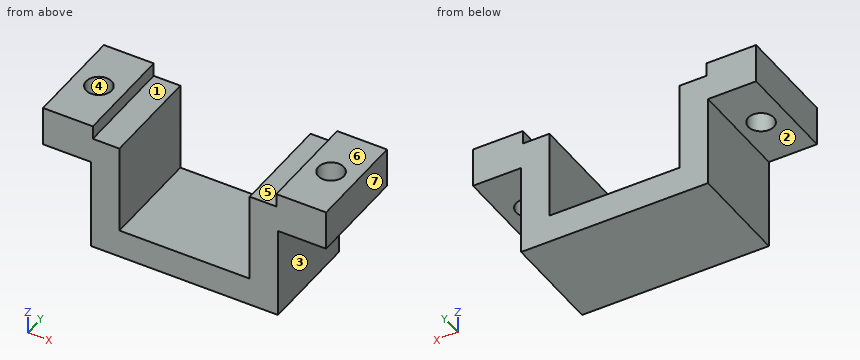
```python
from build123d import *

# Parameters (mm, degrees)
BOSS_EXTRUDE1_DEPTH = 18
SKETCH2_R           = 2.25
CUT_EXTRUDE1_DEPTH  = 56.555737777


with BuildPart() as part:
    # Sketch1 → Boss-Extrude1 (new body)
    with BuildSketch(Plane(origin=(0, 0, 0), x_dir=(1, 0, 0), z_dir=(0, 1, 0))):
        Polygon((0, 0), (8.8, 0), (8.8, 2.4), (13.5, 2.4), (13.5, 18.2), (36.5, 18.2), (36.5, 2.4), (41.2, 2.4), (41.2, 0), (50, 0), (50, 7), (41.5, 7), (41.5, 23.2), (8.5, 23.2), (8.5, 7), (0, 7), align=None)
    extrude(amount=BOSS_EXTRUDE1_DEPTH)

    # Sketch2 → Cut-Extrude1 (cut, through all)
    with BuildSketch(Plane(origin=(0, 0, -7), x_dir=(-1, 0, 0), z_dir=(0, 0, -1))):
        with Locations((-45.5, 9)):
            Circle(SKETCH2_R)
        with Locations(Location((-4.5, 9, 0), (0, 0, 180))):
            Circle(SKETCH2_R)
    extrude(amount=-CUT_EXTRUDE1_DEPTH, mode=Mode.SUBTRACT)


solid = part.part
```
Input: part model. Units: mm. Frame: model coordinates. Face numbers are marked on the shaded views. A direction names the side the tool comes from. Round coordinates to 2 decimals unless told otherwise and drop trailing zeros. Loops run counter-clockwise (first coordinate to the right, second up) from the corner with the lowest first, then second, coordinate; pieces in that order, holes last. Notation, with made-up numbers: (53, 7.5) -> (108, 7.5) arc R12 ccw to (108, 28.5) -> close; hole circle Ø7 at (55, -30). An arc over 180 degrees is marked (long way). Use one line per item in the form item = value. Start each with the question number.
Item 1: Section query B-B on x = 4.5. Return the cut outline in (y, z), then the cut area to 3 significant figures.
Item 2: Material intervals for L1, parallel to Y at x = 4.5, z = -3.5; L2, parallel to X at y = 12.5, z = -4; L3, parallel to X at y = 10, z = -12.25, sorted ascending. Write a range as from..to.
Item 3: Section query C-C on y = 9. Return the cut outline in (x, z).
Item 4: Section query D-D on y = 13.25. Return the cut outline in (x, z), then the cut area to 3 significant figures.
Item 5: Contact query for flat-ended pins moving along their axis: pin 1 Ø4 at (x, y) = (44.5, 11.5) entering from -Z; pin 2 Ø5 at (y, z) = (2.5, -15.5) entering from +X; pin 3 Ø8 at (y, z) = (12, -19) entering from -X. Output: stop coordinate, or through.
Item 6: Mould query, pull axis X, two halves, no side actions, for the marked faces 4, 5, 6 and 7. Classes: pulls with the +X half, pulls with the -X half, needs draft (parallel to the pull), parting line crosses it, or undercut.
Item 7: Section query A-A on z = -15. Return the cut outline in (x, y), then the cut area to 3 significant figures.
Item 8: Set-up query: the marked faces 1, 2 and 3. Return all of +Z, -Z, +X, -X, +Y, -Y with unobstructed straight access to the full face (end or side cutting, diameter ignored); none if empty.
Ans:
q1.outline = (0, -7) -> (6.75, -7) -> (6.75, 0) -> (0, 0) -> close; (11.25, -7) -> (18, -7) -> (18, 0) -> (11.25, 0) -> close
q1.area = 94.5 mm^2
q2.L1 = 0..6.75, 11.25..18
q2.L2 = 0..13.5, 36.5..50
q2.L3 = 8.5..13.5, 36.5..41.5
q3.outline = (0, -7) -> (2.25, -7) -> (2.25, 0) -> (0, 0) -> close; (6.75, -7) -> (8.5, -7) -> (8.5, -23.2) -> (41.5, -23.2) -> (41.5, -7) -> (43.25, -7) -> (43.25, 0) -> (41.2, 0) -> (41.2, -2.4) -> (36.5, -2.4) -> (36.5, -18.2) -> (13.5, -18.2) -> (13.5, -2.4) -> (8.8, -2.4) -> (8.8, 0) -> (6.75, 0) -> close; (47.75, -7) -> (50, -7) -> (50, 0) -> (47.75, 0) -> close
q4.outline = (0, -7) -> (8.5, -7) -> (8.5, -23.2) -> (41.5, -23.2) -> (41.5, -7) -> (50, -7) -> (50, 0) -> (41.2, 0) -> (41.2, -2.4) -> (36.5, -2.4) -> (36.5, -18.2) -> (13.5, -18.2) -> (13.5, -2.4) -> (8.8, -2.4) -> (8.8, 0) -> (0, 0) -> close
q4.area = 443 mm^2
q5.pin_1 = -7
q5.pin_2 = 41.5
q5.pin_3 = 8.5
q6.face_4 = undercut
q6.face_5 = undercut
q6.face_6 = needs draft
q6.face_7 = pulls with the +X half
q7.outline = (8.5, 0) -> (13.5, 0) -> (13.5, 18) -> (8.5, 18) -> close; (36.5, 0) -> (41.5, 0) -> (41.5, 18) -> (36.5, 18) -> close
q7.area = 180 mm^2
q8.face_1 = +Z, +Y, -Y
q8.face_2 = -Z, -X, +Y, -Y
q8.face_3 = -Z, +X, +Y, -Y
